Geometry: see drawing. Coordinates: mm, zero at the bounding-box minimum. Coordinates: 2 decimals unless noted, no trailing zeros. Write each loop counter-clockwise with the first axis right and the second up, starting at its lowest first coordinate (ties: lowest second). Pieces come first, ordered by that corner, then holes. Notation, with made-up numbers: M -1.5,68.25 L 7.5,68.25 A30 ccw 7.5,102.25 Z; hole C 25.25,-32 d6. An arc over 180 degrees is marked long. One line per item, written item: value. Start each with the question number.
Item 1: Cut plane C-C, the plane z = 1.15. Output: boundary loops of the cut face in (x, y).
Item 2: Cut plane A-A, the plane y = 7.8. Output: boundary loops of the cut face in (x, z), then the cut area to 3 significant figures.
Item 3: Mould query, pull axis X, two halves, no side actions, for the marked faces 1, 2 and 3. Classes: released by +X, released by -X, zero draft, split by the parting line, or undercut.
Item 4: Ray query, L1, parallel to Y at x = 7.8, z = 1.45; L2, parallel to X at y = 10.5, z = 1.6; L3, parallel to Z at x = 12.25, y = 13.5. Return the intervals inside material, ascending. Write a range as from..to.
Item 5: Pin query (flat end, axial travel): P1, Ø2, axis at x = 9, z = 0.5, coming from the -Y side; P2, Ø2, axis at y = 11.5, z = 2, coming from the +X side. Return the tip coordinate at first contact, or that it passes through.
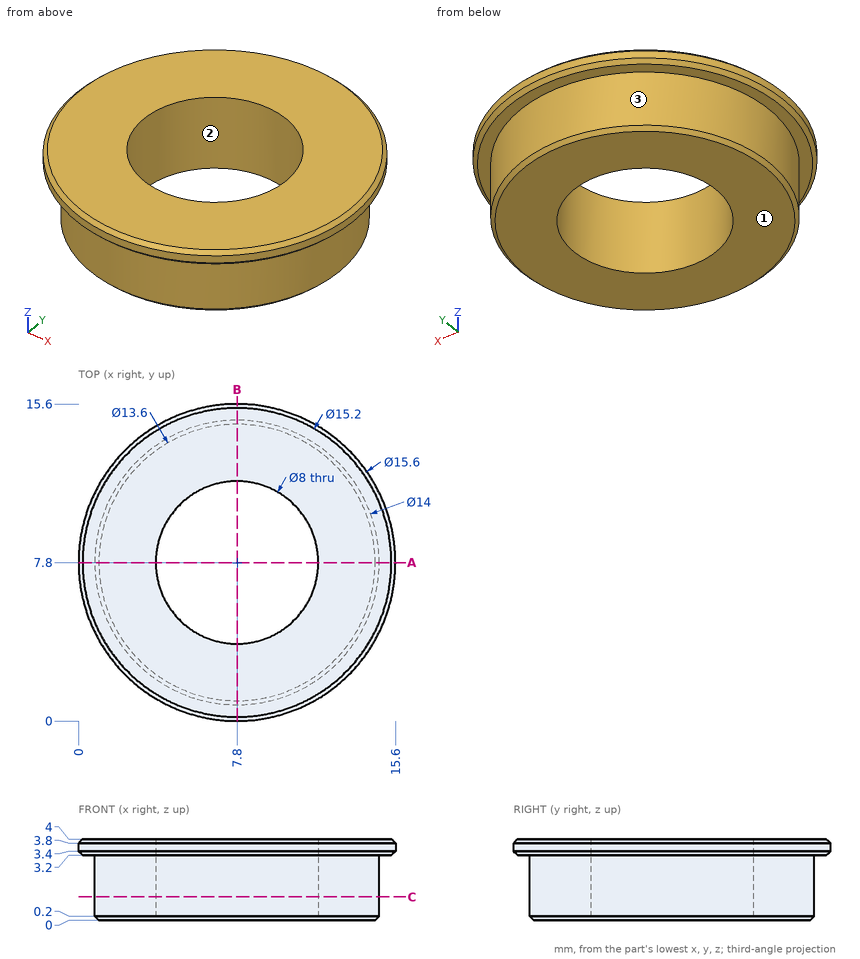
From the geometry:
1. outline: C 7.8,7.8 d14; hole C 7.8,7.8 d8
2. outline: M 0,3.4 L 0.2,3.2 L 0.8,3.2 L 0.8,0.2 L 1,0 L 3.8,0 L 3.8,4 L 0.2,4 L 0,3.8 Z; M 11.8,0 L 14.6,0 L 14.8,0.2 L 14.8,3.2 L 15.4,3.2 L 15.6,3.4 L 15.6,3.8 L 15.4,4 L 11.8,4 Z
2. area: 25.2 mm²
3. face 1: zero draft
3. face 2: undercut
3. face 3: split by the parting line
4. L1: y = 0.8..3.8, 11.8..14.8
4. L2: x = 1.34..4.85, 10.75..14.26
4. L3: z = 3.2..4
5. P1: stops at y = 0.8
5. P2: stops at x = 14.26
